Here's how the part is built. I have some questions about the finished solid (model axes, mm). A direction names the side the tool comes from. Give positions to 0.01 mm unless a question says otherwise; leave off trailing zeros. Order: outer loops, then holes, each group sorted by start corner. A loop starts at its lowest first (then second) coordinate and runs counter-clockwise, first axis right, second up. Notation, with made-up numbers: (-8, -19) - (41, -19) arc R26 cw to (41, -5) - close; hole circle Ø8 at (-36, 82). An arc over 180 degrees is marked (long way). One line per question, with ' | ' between items.
from build123d import *
from build123d.topology import SkipClean

# Parameters (mm, degrees)
SKETCH1_W               = 35
SKETCH1_H               = 35
BOSS_EXTRUDE1_DEPTH     = 8
BOSS_EXTRUDE2_DEPTH     = 12
M18_CLEARANCE_HOLE1_D   = 20
SKETCH5_W               = 3.3
SKETCH5_H               = 8
CUT_EXTRUDE1_DEPTH      = 28.504545079
MIRROR5_COPY_1_SKETCH_W = 3.3
MIRROR5_COPY_1_SKETCH_H = 8
CUT_EXTRUDE2_DEPTH      = 28.504545079


with BuildPart() as part:
    # Sketch1 → Boss-Extrude1 (new body)
    # profile 1 of 2: a face of its own
    with BuildSketch(Plane(origin=(0, 0, 0), x_dir=(1, 0, 0), z_dir=(0, 1, 0))):
        Rectangle(SKETCH1_W, SKETCH1_H)
        Polygon((-6.834523779, -16.5), (6.834523779, -16.5), (16.5, -6.834523779), (16.5, 6.834523779), (6.834523779, 16.5), (-6.834523779, 16.5), (-16.5, 6.834523779), (-16.5, -6.834523779), align=None, mode=Mode.SUBTRACT)
    # profile 2 of 2: a face of its own
    with BuildSketch(Plane(origin=(0, 0, 0), x_dir=(1, 0, 0), z_dir=(0, 1, 0))):
        Polygon((-16.5, -6.834523779), (-6.834523779, -16.5), (6.834523779, -16.5), (16.5, -6.834523779), (16.5, 6.834523779), (6.834523779, 16.5), (-6.834523779, 16.5), (-16.5, 6.834523779), align=None)
    extrude(amount=-BOSS_EXTRUDE1_DEPTH)

    # Sketch1_3 → Boss-Extrude2 (add)
    with BuildSketch(Plane(origin=(0, 0, 0), x_dir=(1, 0, 0), z_dir=(0, 1, 0))):
        Polygon((-16.5, -6.834523779), (-6.834523779, -16.5), (6.834523779, -16.5), (16.5, -6.834523779), (16.5, 6.834523779), (6.834523779, 16.5), (-6.834523779, 16.5), (-16.5, 6.834523779), align=None)
    extrude(amount=BOSS_EXTRUDE2_DEPTH)

    # M18 Clearance Hole1 (through all)
    with Locations(Plane(origin=(0, 12, 0), x_dir=(1, 0, 0), z_dir=(0, 1, 0))):
        with Locations((0, 0)):
            Hole(M18_CLEARANCE_HOLE1_D / 2)

    # Sketch5 → M6 Clearance Hole1 (revolve, cut)
    with BuildSketch(Plane(origin=(-12.5, 0, -12.5), x_dir=(0, 0, 1), z_dir=(1, 0, 0))):
        with Locations((1.65, 4)):
            Rectangle(SKETCH5_W, SKETCH5_H)
    m6_clearance_hole1 = revolve(axis=Axis((-12.5, 6.35, -12.5), (0, -1, 0)), mode=Mode.SUBTRACT)

    # Sketch6 → Cut-Extrude1 (cut, through all)
    with SkipClean():  # the faces are left unmerged after this step: merging them gives an invalid solid
        with BuildSketch(Plane.XZ):
            with BuildLine():
                Line((-13.847066294, -9.487457486), (-9.487457486, -13.847066294))
                ThreePointArc((-9.487457486, -13.847066294), (-10.166547622, -10.166547622), (-13.847066294, -9.487457486))
            make_face()
        extrude(amount=-CUT_EXTRUDE1_DEPTH, mode=Mode.SUBTRACT)

    # Mirror4: M6 Clearance Hole1 across plane
    with SkipClean():  # the faces are left unmerged after this step: merging them gives an invalid solid
        add(m6_clearance_hole1.mirror(Plane(origin=(0, 0, 0), x_dir=(0, 0, 1), z_dir=(1, 0, 0))), mode=Mode.SUBTRACT)

    # Mirror5: M6 Clearance Hole1 across plane
    with SkipClean():  # the faces are left unmerged after this step: merging them gives an invalid solid
        add(m6_clearance_hole1.mirror(Plane.XY), mode=Mode.SUBTRACT)

    # Mirror5 copy 1 sketch → Mirror5 copy 1 (revolve, cut)
    with SkipClean():  # the faces are left unmerged after this step: merging them gives an invalid solid
        with BuildSketch(Plane(origin=(12.5, 0, 12.5), x_dir=(0, 0, -1), z_dir=(-1, 0, 0))):
            with Locations((1.65, 4)):
                Rectangle(MIRROR5_COPY_1_SKETCH_W, MIRROR5_COPY_1_SKETCH_H)
        revolve(axis=Axis((12.5, 6.35, 12.5), (0, -1, 0)), mode=Mode.SUBTRACT)

    # Sketch7 → Cut-Extrude2 (cut, through all)
    with SkipClean():  # the faces are left unmerged after this step: merging them gives an invalid solid
        with BuildSketch(Plane.XZ):
            with BuildLine():
                Line((-9.487457486, 13.847066294), (-13.847066294, 9.487457486))
                ThreePointArc((-13.847066294, 9.487457486), (-10.166547622, 10.166547622), (-9.487457486, 13.847066294))
            make_face()
            with BuildLine():
                Line((13.847066294, 9.487457486), (9.487457486, 13.847066294))
                ThreePointArc((9.487457486, 13.847066294), (10.166547622, 10.166547622), (13.847066294, 9.487457486))
            make_face()
            with BuildLine():
                Line((9.487457486, -13.847066294), (13.847066294, -9.487457486))
                ThreePointArc((13.847066294, -9.487457486), (10.166547622, -10.166547622), (9.487457486, -13.847066294))
            make_face()
        extrude(amount=-CUT_EXTRUDE2_DEPTH, mode=Mode.SUBTRACT)


solid = part.part
1) Please list where these lines run through material, in increasing order: L1, parallel to Z at x = -12.5, y = -6.25; L2, parallel to Z at x = 11, y = -4.75.
Model answer:
L1: z = -17.5 to -15.8, -9.2 to 9.2, 15.8 to 17.5 | L2: z = -17.5 to -15.44, -9.56 to 9.56, 15.44 to 17.5
2) On a 3-axis mill with a long thin cutter (end or side, diameter ignored), from which of +Z, -Z, +X, -X, +Y, -Y can I reach the whole of each face in a straight line? I mean faces 4 (the face through (8.18, 5.916, -15.155)), 5 (the face through (8.142, 5.916, 15.192)), 6 (the face through (-15.155, 5.916, -8.18)), 7 (the face through (-16.5, 6, 0)). Say none if no direction works.
Model answer:
face 4: -Z, +X, +Y | face 5: +Z, +X, +Y | face 6: -Z, -X, +Y | face 7: +Z, -Z, -X, +Y
3) I want a section at B-B (y = -3). List the corners of the cut face in (x, z) for me.
Model answer:
outline: (-17.5, -17.5) - (17.5, -17.5) - (17.5, 17.5) - (-17.5, 17.5) - close; hole circle Ø6.6 at (-12.5, -12.5); hole circle Ø6.6 at (-12.5, 12.5); hole circle Ø20 at (0, 0); hole circle Ø6.6 at (12.5, -12.5); hole circle Ø6.6 at (12.5, 12.5)
4) I want a section at D-D (y = 9). List the corners of the cut face in (x, z) for me, plus the area to 3 significant figures.
Model answer:
outline: (-16.5, -6.83) - (-13.85, -9.49) arc R3.3 cw to (-9.49, -13.85) - (-6.83, -16.5) - (6.83, -16.5) - (9.49, -13.85) arc R3.3 cw to (13.85, -9.49) - (16.5, -6.83) - (16.5, 6.83) - (13.85, 9.49) arc R3.3 cw to (9.49, 13.85) - (6.83, 16.5) - (-6.83, 16.5) - (-9.49, 13.85) arc R3.3 cw to (-13.85, 9.49) - (-16.5, 6.83) - close; hole circle Ø20 at (0, 0) | area: 550 mm2
5) I want a section at A-A (x = 6). List the corners of the cut face in (y, z) for me, plus the area to 3 significant figures.
Model answer:
outline: (-8, -17.5) - (0, -17.5) - (0, -16.5) - (12, -16.5) - (12, -8) - (-8, -8) - close; (-8, 8) - (12, 8) - (12, 16.5) - (0, 16.5) - (0, 17.5) - (-8, 17.5) - close | area: 356 mm2
6) Thinking about a two-plate mould opening in X: for faces 1 (the face through (-8.142, 5.916, -15.192)), 2 (the face through (2.17, 1.86, 9.76)), 3 (the face through (16.5, 6, 0)), which applies, +X half, -X half, draft (parallel to the pull), parting line (faces both ways), or undercut?
Model answer:
face 1: -X half | face 2: undercut | face 3: +X half
7) I want a section at C-C (z = 12.5). List the corners of the cut face in (x, y) for me, plus the area to 3 significant figures.
Model answer:
outline: (-17.5, -8) - (-15.8, -8) - (-15.8, 0) - (-17.5, 0) - close; (-9.2, -8) - (9.2, -8) - (9.2, 12) - (-9.2, 12) - close; (15.8, -8) - (17.5, -8) - (17.5, 0) - (15.8, 0) - close | area: 395 mm2
8) I'm going to push flat-ended pins straight in: P1, Ø10, axis at y = 7.5, z = -1, coming from the -X side; P2, Ø8, axis at x = 8, y = 9.5, coming from the +Z side; P3, Ø3.5, axis at y = 6, z = 0.5, coming from the +X side. Where does each tip first touch, or does it pass through?
Model answer:
P1: stops at x = -16.5 | P2: stops at z = 16.5 | P3: stops at x = 16.5
